from build123d import *

# Parameters (mm, degrees)
BOSS_EXTRU_1_DEPTH         = 2960
ESQUISSE7_R                = 6
ENL_V_MAT_EXTRU_2_DEPTH    = 2962.718746921
ESQUISSE8_W                = 40
ESQUISSE8_H                = 100
ENL_V_MAT_EXTRU_3_DEPTH    = 2962.718746921
R_P_TITION_LIN_AIRE1_COUNT = 24
R_P_TITION_LIN_AIRE1_PITCH = 310
ESQUISSE9_R                = 27
ENL_V_MAT_EXTRU_4_DEPTH    = 2962.77126058


with BuildPart() as part:
    # Esquisse1 → Boss.-Extru.1 (new body)
    with BuildSketch(Plane.XY):
        Polygon((-3.600291477, 0), (36.399708523, 0), (36.399708523, 5), (1.399708523, 5), (1.399708523, 87), (41.399708523, 87), (41.399708523, 92), (-3.600291477, 92), align=None)
    extrude(amount=BOSS_EXTRU_1_DEPTH)

    # Esquisse7 → Enlèv. mat.-Extru.2 (cut, through all)
    with BuildSketch(Plane(origin=(0, 92, 0), x_dir=(1, 0, 0), z_dir=(0, 1, 0))):
        with Locations(Location((21.399708523, -135, 0), (0, 0, 180))):
            Circle(ESQUISSE7_R)
    enl_v_mat_extru_2 = extrude(amount=-ENL_V_MAT_EXTRU_2_DEPTH, mode=Mode.SUBTRACT)

    # Esquisse8 → Enlèv. mat.-Extru.3 (cut, through all)
    with BuildSketch(Plane(origin=(0, 92, 0), x_dir=(1, 0, 0), z_dir=(0, 1, 0))):
        with Locations((21.399708523, -2910)):
            Rectangle(ESQUISSE8_W, ESQUISSE8_H)
        with Locations((21.399708523, -50)):
            Rectangle(ESQUISSE8_W, ESQUISSE8_H)
    extrude(amount=-ENL_V_MAT_EXTRU_3_DEPTH, mode=Mode.SUBTRACT)

    # Répétition linéaire1: Enlèv. mat.-Extru.2 ×24
    with Locations(*[(0, 0, i * R_P_TITION_LIN_AIRE1_PITCH) for i in range(1, R_P_TITION_LIN_AIRE1_COUNT)]):
        add(enl_v_mat_extru_2, mode=Mode.SUBTRACT)

    # Esquisse9 → Enlèv. mat.-Extru.4 (cut, through all)
    with BuildSketch(Plane.ZY.offset(3.600291477)):
        with Locations(Location((55, 46, 0), (0, 0, 270))):
            Circle(ESQUISSE9_R)
        with Locations(Location((2905, 46, 0), (0, 0, 270))):
            Circle(ESQUISSE9_R)
    extrude(amount=-ENL_V_MAT_EXTRU_4_DEPTH, mode=Mode.SUBTRACT)


solid = part.part
Here's how the part is built. I have some questions about the finished solid (model axes, mm). Coordinates: 2 decimals unless noted, no trailing zeros. Order: outer loops, then holes, each group sorted by start corner. A loop starts at its lowest first (then second) coordinate and runs counter-clockwise, first axis right, second up. Notation, with made-up numbers: (55.5, 89.5) -> (109.5, 89.5) arc R22 cw to (109.5, 97.5) -> close; hole circle Ø9 at (12, 17.25). An arc over 180 degrees is marked (long way). Answer in a Markdown table with one row per item.
(1) Please list where these lines run through material, in increasing order: probe 1 along Y at (x, z) = (5, 1700); probe 2 along X at (y, z) = (3.85, 1685); probe 3 along Z at (x, y) = (36, 4.5).
Answer key:
| item | result |
|---|---|
| probe 1 | 0 to 5, 87 to 92 |
| probe 2 | -3.6 to 15.4, 27.4 to 36.4 |
| probe 3 | 100 to 2860 |
(2) I want a section at C-C on z = 2565. List the corners of the cut face in (x, y) for me, then the cut area to 3 significant figures.
Answer key:
| item | result |
|---|---|
| outline | (-3.6, 0) -> (36.4, 0) -> (36.4, 5) -> (1.4, 5) -> (1.4, 87) -> (41.4, 87) -> (41.4, 92) -> (-3.6, 92) -> close |
| area | 835 mm^2 |
(3) I want a section at B-B on z = 55. List the corners of the cut face in (x, y) for me.
Answer key:
| item | result |
|---|---|
| outline | (-3.6, 0) -> (1.4, 0) -> (1.4, 19) -> (-3.6, 19) -> close; (-3.6, 73) -> (1.4, 73) -> (1.4, 92) -> (-3.6, 92) -> close |
(4) Will these pins go through, and if not, where does the flat tip stop? pin 1 Ø7 at (x, z) = (21.4, 1375) entering from -Y; pin 2 Ø2.5 at (x, y) = (11.5, 88.5) entering from +Z; pin 3 Ø4 at (y, z) = (10.5, 1340) entering from +X; pin 4 Ø1.5 at (y, z) = (2.5, 1713.5) entering from +X.
Answer key:
| item | result |
|---|---|
| pin 1 | through |
| pin 2 | z = 2860 |
| pin 3 | x = 1.4 |
| pin 4 | x = 36.4 |
(5) I want a section at A-A on y = 43. List the corners of the cut face in (x, z) for me, then the cut area to 3 significant figures.
Answer key:
| item | result |
|---|---|
| outline | (-3.6, 0) -> (1.4, 0) -> (1.4, 28.17) -> (-3.6, 28.17) -> close; (-3.6, 81.83) -> (1.4, 81.83) -> (1.4, 2878.17) -> (-3.6, 2878.17) -> close; (-3.6, 2931.83) -> (1.4, 2931.83) -> (1.4, 2960) -> (-3.6, 2960) -> close |
| area | 14,300 mm^2 |
(6) Thinking about a two-plate mould opening in Y: for faces 1 (the face through (19, 92, 1459)), 2 (the face through (1.4, 36, 1501)), 3 (the face through (-3.6, 47, 1459)), 4 (the face through (-1.14, 21.06, 44.66)), which applies, +Y half, -Y half, draft (parallel to the pull), parting line (faces both ways), or undercut?
Answer key:
| item | result |
|---|---|
| face 1 | +Y half |
| face 2 | undercut |
| face 3 | draft |
| face 4 | undercut |
